The listing builds one solid part. Answer for the finished solid, in the listing's coordinates (mm). Face numbers are marked on the shaded views. A direction names the side the tool comes from. Coordinates: 2 decimals unless noted, no trailing zeros. Order: outer loops, then holes, each group sorted by start corner. A loop starts at its lowest first (then second) coordinate and runs counter-clockwise, first axis right, second up. Notation, with made-up numbers: (83, 3) -> (100, 3) arc R20 ccw to (100, 41) -> close; hole circle Ø11 at (-28, 73). An arc over 180 degrees is marked (long way). Write each question's results on one line, items separated by ' | '. Start each with the question number.
(1) The part is cut by section A-A, the plane y = -5. Give the vertices of the cut face in (x, z), then the cut area to 3 significant figures.
(2) Given pin 1 (1.8 mm diameter, centred on x = -46.5, y = -1.25, fed in from +Z); pin 2 (2 mm diameter, centred on x = -33.5, y = -14, fed in from +Z); pin 3 (3 mm diameter, centred on x = -34.5, z = -38.5, fed in from -Y), each flat-ended and moving along its own axis, determine where each tip first touches the part or whether it passes through.
(3) Straight lines are drawn through the part: L1, parallel to X at y = -10, z = -46; L2, parallel to X at y = 32, z = 7; L3, parallel to X at y = -18, z = -46. For each, find the intervals that lie inside material, in ascending order.
(4) A tool of negligible diameter and unlimited length cuts with its end or side. For the marked faces 1 and 2, from which of +Z, -Z, +X, -X, +Y, -Y can it reach the whole face along a straight path? Write none if from no direction.
(5) The part is cut by section B-B, the plane z = 7.5. Give the vertices of the cut face in (x, y), then the cut area to 3 significant figures.
(6) The part is cut by section D-D, the plane z = -35.5. Give the vertices of the cut face in (x, y).
(7) The part is cut by section C-C, the plane x = -43. Give the vertices of the cut face in (y, z).
```python
from build123d import *

# Parameters (mm, degrees)
SKETCH1_W           = 120
SKETCH1_H           = 60
SKETCH1_R           = 1
SKETCH1_W_2         = 22
SKETCH1_H_2         = 44
SKETCH1_H_3         = 20
BOSS_EXTRUDE1_DEPTH = 35
CUT_EXTRUDE1_REACH  = 171.853
SKETCH2_W           = 75
SKETCH2_H           = 65
SKETCH3_W           = 40
SKETCH3_H           = 65
CUT_EXTRUDE2_DEPTH  = 5
FILLET1_R           = 5
SKETCH4_R           = 1
CUT_EXTRUDE3_DEPTH  = 5


with BuildPart() as part:
    # Sketch1 → Boss-Extrude1 (new, symmetric)
    # profile 1 of 2: a face of its own
    with BuildSketch(Plane(origin=(0, 0, 0), x_dir=(1, 0, 0), z_dir=(0, 1, 0))):
        Rectangle(SKETCH1_W, SKETCH1_H)
        with Locations(Location((-4.85, -24, 0), (0, 0, 270))):
            Circle(SKETCH1_R, mode=Mode.SUBTRACT)
        Rectangle(SKETCH1_W_2, SKETCH1_H_2, mode=Mode.SUBTRACT)
        with Locations(Location((4.85, -24, 0), (0, 0, 270))):
            Circle(SKETCH1_R, mode=Mode.SUBTRACT)
        with Locations(Location((-4.85, 24, 0), (0, 0, 270))):
            Circle(SKETCH1_R, mode=Mode.SUBTRACT)
        with Locations(Location((4.85, 24, 0), (0, 0, 270))):
            Circle(SKETCH1_R, mode=Mode.SUBTRACT)
    # profile 2 of 2: a face of its own
    with BuildSketch(Plane(origin=(0, 0, 0), x_dir=(1, 0, 0), z_dir=(0, 1, 0))):
        with Locations((0, 40)):
            Rectangle(SKETCH1_W, SKETCH1_H_3)
    extrude(amount=BOSS_EXTRUDE1_DEPTH, both=True)

    # Cut-Extrude1: up to this face of the body (flat: up to its plane)
    cut_extrude1_end = Plane(part.part.faces().sort_by_distance((60, 0, -10))[0])
    # Sketch2 → Cut-Extrude1 (cut, up to the picked face)
    with BuildSketch(Plane(origin=(-60, 0, -85), x_dir=(0, 0, -1), z_dir=(1, 0, 0)), mode=Mode.PRIVATE) as cut_extrude1_sk1:
        with Locations((-77.5, -2.5)):
            Rectangle(SKETCH2_W, SKETCH2_H)
    cut_extrude1_tool1 = split(extrude(cut_extrude1_sk1.sketch, amount=CUT_EXTRUDE1_REACH, mode=Mode.PRIVATE), bisect_by=cut_extrude1_end, keep=Keep.BOTH, mode=Mode.PRIVATE)
    add(cut_extrude1_tool1.solids().sort_by(Axis((-60, -2.5, -7.5), (1, 0, 0)))[0], mode=Mode.SUBTRACT)

    # Sketch3 → Cut-Extrude2 (cut)
    with BuildSketch(Plane(origin=(0, 0, -50), x_dir=(-1, 0, 0), z_dir=(0, 0, -1))):
        with Locations((0, -2.5)):
            Rectangle(SKETCH3_W, SKETCH3_H)
    extrude(amount=-CUT_EXTRUDE2_DEPTH, mode=Mode.SUBTRACT)

    # Fillet1
    fillet1_edges = [part.edges().sort_by_distance(p)[0] for p in [
        (40, 30, -45),
        (-40, 30, -45),
        (-20, 30, -47.5),
        (20, 30, -47.5),
    ]]
    fillet(fillet1_edges, radius=FILLET1_R)

    # Sketch4 → Cut-Extrude3 (cut)
    with BuildSketch(Plane.XY.offset(-45)):
        with Locations((-40, -18.5)):
            Circle(SKETCH4_R)
        with Locations((-40, -15.5)):
            Circle(SKETCH4_R)
        with Locations((-40, -12.5)):
            Circle(SKETCH4_R)
        with Locations((-46.495190528, -8.75)):
            Circle(SKETCH4_R)
        with Locations((-49.09326674, -10.25)):
            Circle(SKETCH4_R)
        with Locations((-51.691342951, -11.75)):
            Circle(SKETCH4_R)
        with Locations((-46.495190528, -1.25)):
            Circle(SKETCH4_R)
        with Locations((-49.09326674, 0.25)):
            Circle(SKETCH4_R)
        with Locations((-51.691342951, 1.75)):
            Circle(SKETCH4_R)
        with Locations((-40, 2.5)):
            Circle(SKETCH4_R)
        with Locations((-40, 5.5)):
            Circle(SKETCH4_R)
        with Locations((-40, 8.5)):
            Circle(SKETCH4_R)
        with Locations((-33.504809472, -1.25)):
            Circle(SKETCH4_R)
        with Locations((-30.90673326, 0.25)):
            Circle(SKETCH4_R)
        with Locations((-28.308657049, 1.75)):
            Circle(SKETCH4_R)
        with Locations((-33.504809472, -8.75)):
            Circle(SKETCH4_R)
        with Locations((-30.90673326, -10.25)):
            Circle(SKETCH4_R)
        with Locations((-28.308657049, -11.75)):
            Circle(SKETCH4_R)
        with Locations((40, -18.5)):
            Circle(SKETCH4_R)
        with Locations((40, -15.5)):
            Circle(SKETCH4_R)
        with Locations((40, -12.5)):
            Circle(SKETCH4_R)
        with Locations((33.504809472, -8.75)):
            Circle(SKETCH4_R)
        with Locations((30.90673326, -10.25)):
            Circle(SKETCH4_R)
        with Locations((28.308657049, -11.75)):
            Circle(SKETCH4_R)
        with Locations((33.504809472, -1.25)):
            Circle(SKETCH4_R)
        with Locations((30.90673326, 0.25)):
            Circle(SKETCH4_R)
        with Locations((28.308657049, 1.75)):
            Circle(SKETCH4_R)
        with Locations((40, 2.5)):
            Circle(SKETCH4_R)
        with Locations((40, 5.5)):
            Circle(SKETCH4_R)
        with Locations((40, 8.5)):
            Circle(SKETCH4_R)
        with Locations((46.495190528, -1.25)):
            Circle(SKETCH4_R)
        with Locations((49.09326674, 0.25)):
            Circle(SKETCH4_R)
        with Locations((51.691342951, 1.75)):
            Circle(SKETCH4_R)
        with Locations((46.495190528, -8.75)):
            Circle(SKETCH4_R)
        with Locations((49.09326674, -10.25)):
            Circle(SKETCH4_R)
        with Locations((51.691342951, -11.75)):
            Circle(SKETCH4_R)
    extrude(amount=-CUT_EXTRUDE3_DEPTH, mode=Mode.SUBTRACT)


solid = part.part
```
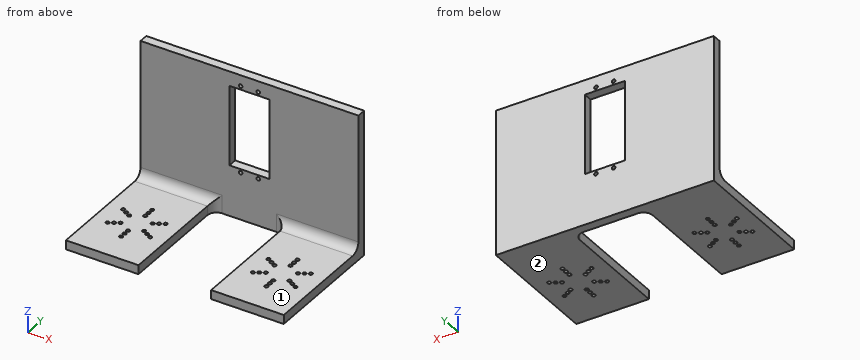
Established:
1) outline: (-60, -50) -> (-20, -50) -> (-20, -45) -> (-60, -45) -> close; (20, -50) -> (60, -50) -> (60, -45) -> (20, -45) -> close | area: 400 mm^2
2) pin 1: passes through | pin 2: stops at z = -45 | pin 3: stops at y = 30
3) L1: x = -60 to -50.06, -48.13 to -31.87, -29.94 to -20, 20 to 29.94, 31.87 to 48.13, 50.06 to 60 | L2: x = -60 to -11, 11 to 60 | L3: x = -60 to -40.87, -39.13 to -20, 20 to 39.13, 40.87 to 60
4) face 1: +Z, +X, -X, -Y | face 2: -Z, +X, -X, +Y, -Y
5) outline: (-60, 30) -> (-11, 30) -> (-11, 35) -> (-60, 35) -> close; (11, 30) -> (60, 30) -> (60, 35) -> (11, 35) -> close | area: 490 mm^2
6) outline: (-60, 30) -> (60, 30) -> (60, 35) -> (-60, 35) -> close
7) outline: (-35, -50) -> (35, -50) -> (35, 30) -> (30, 30) -> (30, -40) arc R5 cw to (25, -45) -> (-35, -45) -> close
